Design review of the part built by this model. Coordinates are the model's own, in mm. Face numbers are marked on the shaded views. A direction names the side the tool comes from. Give positions to 0.01 mm unless a question says otherwise; leave off trailing zeros. Write each loop counter-clockwise with the first axis right and the second up, starting at its lowest first coordinate (ties: lowest second). Pieces come first, ordered by that corner, then holes. Notation, with made-up numbers: (-22, 83.5) -> (-10, 83.5) arc R16 cw to (-10, 95.5) -> close; hole circle Ø2 at (-39, 7.25). An arc over 180 degrees is marked (long way). Answer as a JSON object with one key per item and string values.
```python
from build123d import *

# Parameters (mm, degrees)
F1_DEPTH = 21
F2_W     = 41
F2_H     = 57
F3_DEPTH = 5
F4_W     = 41
F4_H     = 49
F5_DEPTH = 5
F7_DEPTH = 5


with BuildPart() as f1:
    # F0 (on Right) → F1 (new body)
    with BuildSketch(Plane.YZ):
        Polygon((15.559513, 19), (15.559513, 0), (-15.440487, 0), (-15.440487, 19), (-20.440487, 19), (-20.440487, 0), (-20.440487, -38), (-15.440487, -38), (15.469343, -38), (20.559513, -38), (20.559513, 0), (20.559513, 19), align=None)
    extrude(amount=F1_DEPTH)

    # F2 (on face) → F3 (join)
    with BuildSketch(Plane.YZ.offset(21)):
        with Locations((0.059513, -9.5)):
            Rectangle(F2_W, F2_H)
    extrude(amount=F3_DEPTH)

    # F4 (on face) → F5 (join)
    with BuildSketch(Plane(origin=(0, 0, 0), x_dir=(0, -1, 0), z_dir=(-1, 0, 0))):
        with Locations((-0.059513, -13.5)):
            Rectangle(F4_W, F4_H)
    extrude(amount=F5_DEPTH)

    # F6 (on face) → F7 (cut)
    with BuildSketch(Plane(origin=(0, 20.559513, 0), x_dir=(-1, 0, 0), z_dir=(0, 1, 0))):
        with BuildLine():
            Line((-8, 8.489112), (-8, 19))
            Line((-8, 19), (-13, 19))
            Line((-13, 19), (-13, 8.489112))
            ThreePointArc((-13, 8.489112), (-10.5, 5.989112), (-8, 8.489112))
        make_face()
    extrude(amount=-F7_DEPTH, mode=Mode.SUBTRACT)


solid = f1.part
```
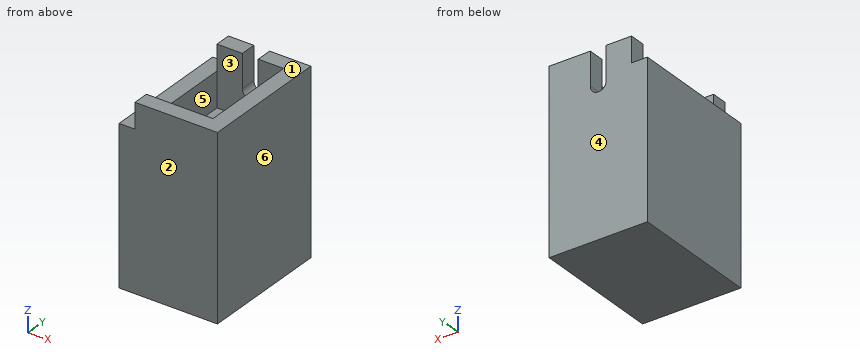
(1) Clearance check with flat-ended pins moving along their axes: pin 1 (2.5 mm diameter, centred on x = -3, y = 2.5, fed in from +Z); pin 2 (1.5 mm diameter, centred on y = 19, z = 15.5, fed in from -X). State where each tip first meets the part, or that it passes through.
Here are the results:
{"pin 1": "stops at z = 11", "pin 2": "stops at x = 0"}
(2) We need section B-B, the plane y = 17. State the section outline as (x, z) points.
Here are the results:
{"outline": "(-5, -38) -> (26, -38) -> (26, 19) -> (13, 19) -> (13, 8.49) arc R2.5 cw to (8, 8.49) -> (8, 19) -> (0, 19) -> (0, 11) -> (-5, 11) -> close"}
(3) We need section C-C, the plane x = 3. State the section outline as (y, z) points, then the cut area to 3 significant figures.
Here are the results:
{"outline": "(-20.44, -38) -> (20.56, -38) -> (20.56, 19) -> (15.56, 19) -> (15.56, 0) -> (-15.44, 0) -> (-15.44, 19) -> (-20.44, 19) -> close", "area": "1,750 mm²"}
(4) We need section D-D, the plane y = -17. State the section outline as (x, z) points.
Here are the results:
{"outline": "(-5, -38) -> (26, -38) -> (26, 19) -> (0, 19) -> (0, 11) -> (-5, 11) -> close"}
(5) For line 1 along Y through (x, z) = (19, 7); line 2 along X through (y, z) = (7.5, 1.5); line 3 along Z through (x, y) = (2, -8), list the stretches that pass through material, from the lowest coordinate up.
Here are the results:
{"line 1": "y = -20.44 to -15.44, 15.56 to 20.56", "line 2": "x = -5 to 0, 21 to 26", "line 3": "z = -38 to 0"}
(6) We need section A-A, the plane z = 12. State the section outline as (x, y) points, then the cut area to 3 significant figures.
Here are the results:
{"outline": "(0, -20.44) -> (26, -20.44) -> (26, 20.56) -> (13, 20.56) -> (13, 15.56) -> (21, 15.56) -> (21, -15.44) -> (0, -15.44) -> close; (0, 15.56) -> (8, 15.56) -> (8, 20.56) -> (0, 20.56) -> close", "area": "390 mm²"}
(7) The part is to be moulded in two halves that separate along Y. For the marked faces 1, 2, 3 and 4, say which applies: +Y half, -Y half, draft (parallel to the pull), parting line (faces both ways), or undercut.
Here are the results:
{"face 1": "draft", "face 2": "-Y half", "face 3": "undercut", "face 4": "+Y half"}
(8) For the marked faces 5 and 6, list the 3-axis set-ups (+Z, -Z, +X, -X, +Y, -Y) from which the entire face can be reached by the end or side of a thin tool; tool diameter is ignored.
Here are the results:
{"face 5": "+Z", "face 6": "+Z, -Z, +X, +Y, -Y"}
